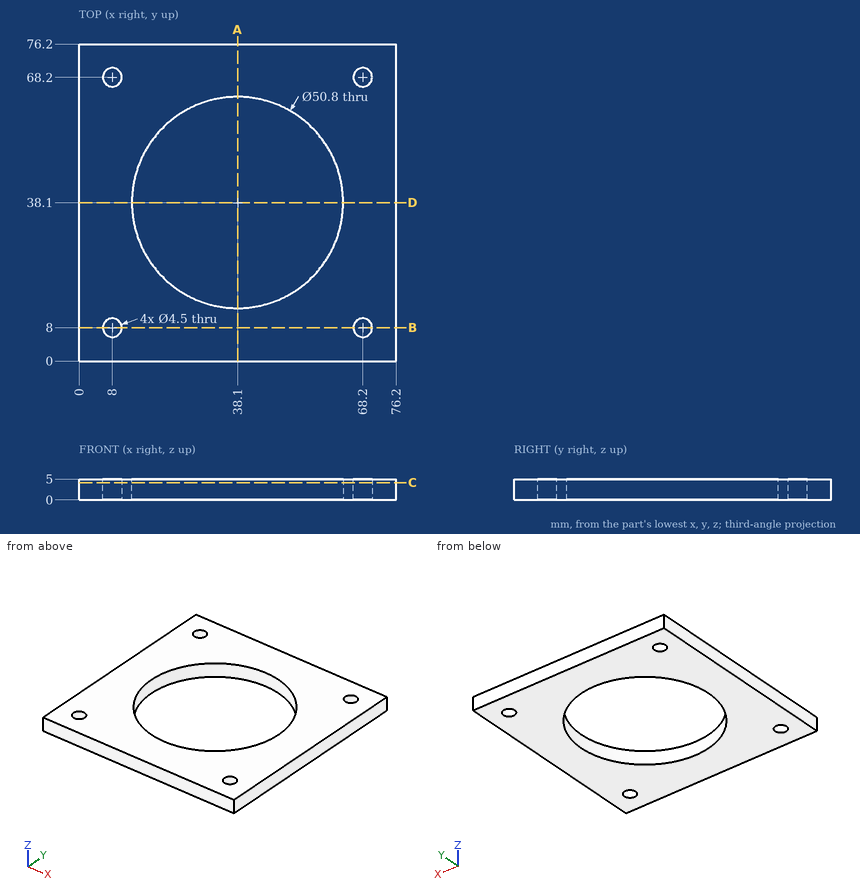
Study the drawing (mm; zero at the part's minimum x, y, z) and answer. Round coordinates to 2 decimals unless told otherwise and drop trailing zeros. Write each loop counter-clockwise with the first axis right and the second up, starting at its lowest first coordinate (ties: lowest second). Pieces come first, ordered by that corner, then holes.
Q1. Find section C-C on z = 4.1. Determine the outline of the cut face in (x, y), and give its area (3 significant figures).
Values:
outline: (0, 0) - (76.2, 0) - (76.2, 76.2) - (0, 76.2) - close; hole circle Ø4.5 at (8, 8); hole circle Ø4.5 at (8, 68.2); hole circle Ø50.8 at (38.1, 38.1); hole circle Ø4.5 at (68.2, 8); hole circle Ø4.5 at (68.2, 68.2)
area: 3,720 mm2
Q2. Find section A-A on x = 38.1. Determine the outline of the cut face in (y, z), and give its area (3 significant figures).
Values:
outline: (0, 0) - (12.7, 0) - (12.7, 5) - (0, 5) - close; (63.5, 0) - (76.2, 0) - (76.2, 5) - (63.5, 5) - close
area: 127 mm2
Q3. Flat-ended cylindrical pins translate along their axes: P1, Ø1.5, axis at x = 21.5, y = 19, coming from the -Z side; P2, Ø4, axis at x = 8, y = 8, coming from the -Z side. Find the tip coordinate at first contact, or state that the pin passes through.
Values:
P1: stops at z = 0
P2: passes through
Q4. Straight lines are drawn through the part: line 1 (Y direction, x = 68.2, z = 3.95); line 2 (Y direction, x = 38.1, z = 3.55); line 3 (Y direction, x = 69, z = 1.4). For each, find the intervals that lie inside material, in ascending order.
Values:
line 1: y = 0 to 5.75, 10.25 to 65.95, 70.45 to 76.2
line 2: y = 0 to 12.7, 63.5 to 76.2
line 3: y = 0 to 5.9, 10.1 to 66.1, 70.3 to 76.2
Q5. Find section B-B on y = 8. Determine the outline of the cut face in (x, z).
Values:
outline: (0, 0) - (5.75, 0) - (5.75, 5) - (0, 5) - close; (10.25, 0) - (65.95, 0) - (65.95, 5) - (10.25, 5) - close; (70.45, 0) - (76.2, 0) - (76.2, 5) - (70.45, 5) - close
